```python
from build123d import *

# Parameters (mm, degrees)
F0_W     = 54.92849
F0_H     = 36.702846
F1_DEPTH = 49.276
F2_R     = 12.902287
F3_DEPTH = 27.94
F4_R     = 9.88166
F5_DEPTH = 92.202


with BuildPart() as f1:
    # F0 (on Front) → F1 (new body)
    with BuildSketch(Plane.XZ):
        Rectangle(F0_W, F0_H)
    extrude(amount=F1_DEPTH)

    # F2 (on Front) → F3 (join)
    with BuildSketch(Plane.XZ):
        Circle(F2_R)
    extrude(amount=-F3_DEPTH)

    # F4 (on face) → F5 (cut)
    with BuildSketch(Plane(origin=(0, 27.94, 0), x_dir=(-1, 0, 0), z_dir=(0, 1, 0))):
        Circle(F4_R)
    extrude(amount=-F5_DEPTH, mode=Mode.SUBTRACT)


solid = f1.part
```
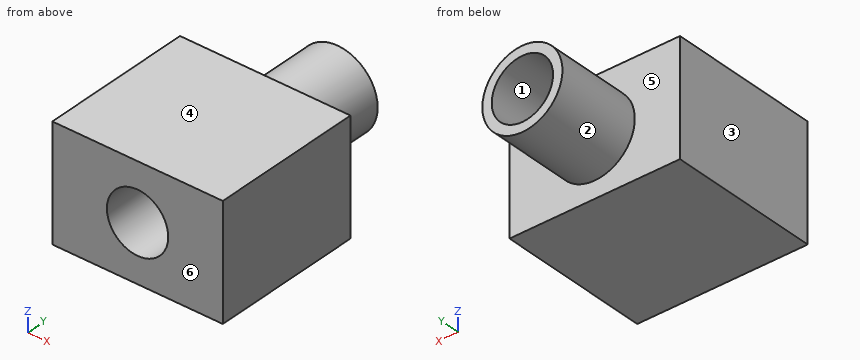
Can you work these out from the model? Positions are in its coordinate system, mm. Face numbers are marked on the shaded views. A direction names the side the tool comes from. Round coordinates to 2 decimals unless told otherwise and drop trailing zeros. Loops run counter-clockwise (first coordinate to the right, second up) from the corner with the lowest first, then second, coordinate; pieces in that order, holes last. Notation, with made-up numbers: M -31,19.5 L 17,19.5 A19 ccw 17,34.5 Z; hole C 30.25,-27 d3. An arc over 180 degrees is marked long. Answer as a JSON object with one key per item and string values. Group by question number.
Q1. We'd pull the mould along Z, two halves only. Please class the marked faces 1, 2, 3 and 4: +Z half, -Z half, draft (parallel to the pull), parting line (faces both ways), or undercut.
Q2. Imagine slicing it at D-D, the plane y = 1. Please give me the cut outline in (x, z), then the cut area to 3 significant figures.
Q3. Please list where these lines run through material, in increasing order: L1, parallel to Z at x = 0, y = -30.5; L2, parallel to Z at x = 0, y = 1; L3, parallel to Y at x = -3, z = 17.5.
Q4. Will these pins go through, and if not, where does the flat tip stop? pin 1 (2 mm diameter, centred on y = 8.5, z = 10.5, fed in from -X); pin 2 (5 mm diameter, centred on x = 10, y = 3, fed in from -Z).
Q5. Imagine slicing it at B-B, the plane z = 0. Please give me the cut outline in (x, y), then the cut area to 3 significant figures.
Q6. On a 3-axis mill with a long thin cutter (end or side, diameter ignored), from which of +Z, -Z, +X, -X, +Y, -Y can I reach the whole of each face in a straight line? I mean the marked faces 5 and 6. Say none if no direction works.
Q7. Imagine slicing it at C-C, the plane y = -26.5. Please give me the cut outline in (x, z).
Q8. Imagine slicing it at A-A, the plane x = 0. Please give me the cut outline in (y, z), then the cut area to 3 significant figures.
Findings:
{
 "1": {"face 1": "undercut", "face 2": "parting line", "face 3": "draft", "face 4": "+Z half"},
 "2": {"outline": "C 0,0 d25.8; hole C 0,0 d19.76", "area": "216 mm2"},
 "3": {"L1": "z = -18.35 to -9.88, 9.88 to 18.35", "L2": "z = -12.9 to -9.88, 9.88 to 12.9", "L3": "y = -49.28 to 0"},
 "4": {"pin 1": "stops at x = -8.73", "pin 2": "stops at z = -10.5"},
 "5": {"outline": "M -27.46,-49.28 L -9.88,-49.28 L -9.88,27.94 L -12.9,27.94 L -12.9,0 L -27.46,0 Z; M 9.88,-49.28 L 27.46,-49.28 L 27.46,0 L 12.9,0 L 12.9,27.94 L 9.88,27.94 Z", "area": "1,900 mm2"},
 "6": {"face 5": "+Y", "face 6": "+Z, -Z, +X, -X, -Y"},
 "7": {"outline": "M -27.46,-18.35 L 27.46,-18.35 L 27.46,18.35 L -27.46,18.35 Z; hole C 0,0 d19.76"},
 "8": {"outline": "M -49.28,-18.35 L 0,-18.35 L 0,-12.9 L 27.94,-12.9 L 27.94,-9.88 L -49.28,-9.88 Z; M -49.28,9.88 L 27.94,9.88 L 27.94,12.9 L 0,12.9 L 0,18.35 L -49.28,18.35 Z", "area": "1,000 mm2"}
}
